Drawing for the job (mm, zero at the part's lowest x, y, z). Give positions to 0.01 mm unless a question says otherwise; leave off trailing zeros. Loops run counter-clockwise (first coordinate to the right, second up) from the corner with the lowest first, then second, coordinate; pieces in that order, holes last. Notation, with made-up numbers: (-20, -5.5) -> (38, -5.5) arc R20 cw to (38, 26.5) -> close; hole circle Ø10 at (6.5, 7). An arc over 180 degrees is marked (long way). Answer in a Markdown table with one row per item. Add a question column.
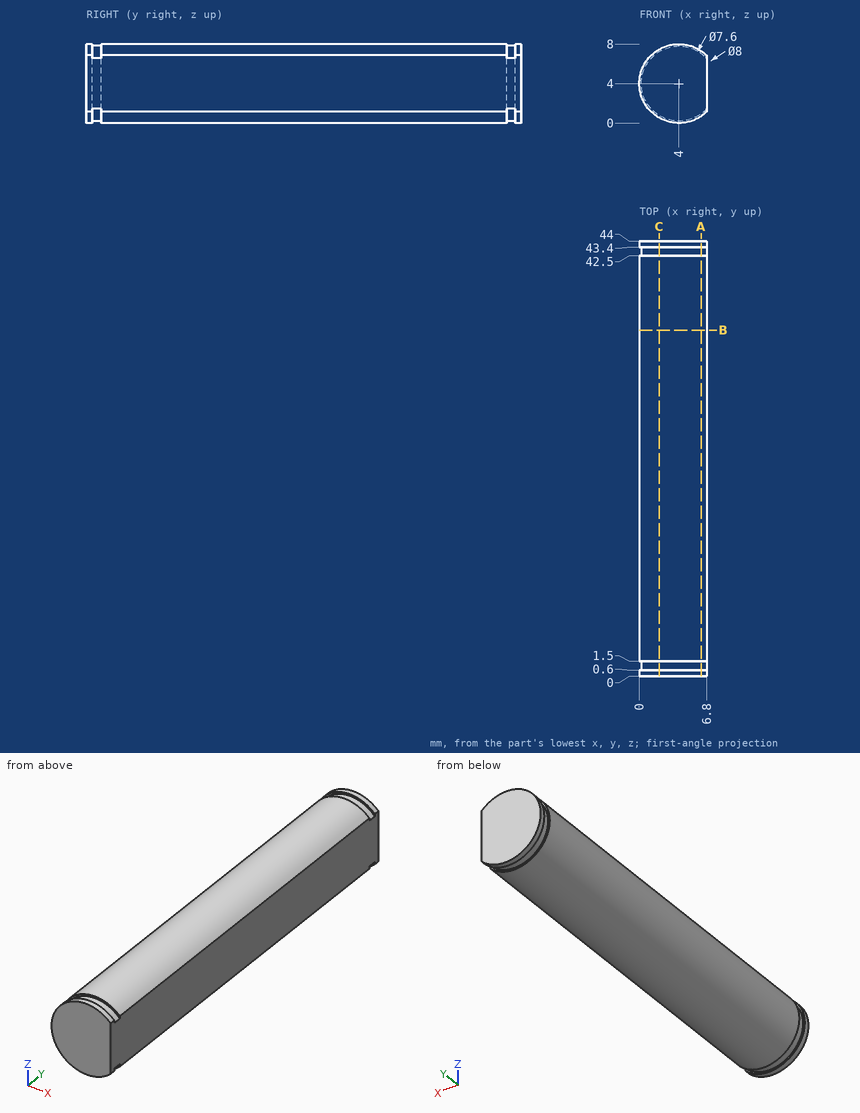
(1) Saw through at C-C, the plane x = 2. List the corners of the cut face in (y, z).
(2) Wall check: line 1 along X through (y, z) = (41.5, 3.75); line 2 along Z through (x, y) = (4.25, 7.5); line 3 along X through (y, z) = (40.5, 2). Give the ranges that are in metal, low to high. Write a range as from..to.
(3) Saw through at A-A, the plane x = 6.25. List the corners of the cut face in (y, z), then the cut area to 3 significant figures.
(4) Saw through at B-B, the plane y = 35. List the corners of the cut face in (x, z), then the cut area to 3 significant figures.
Worked answers:
| question | item | result |
|---|---|---|
| 1 | outline | (0, 0.54) -> (0.6, 0.54) -> (0.6, 0.77) -> (1.5, 0.77) -> (1.5, 0.54) -> (42.5, 0.54) -> (42.5, 0.77) -> (43.4, 0.77) -> (43.4, 0.54) -> (44, 0.54) -> (44, 7.46) -> (43.4, 7.46) -> (43.4, 7.23) -> (42.5, 7.23) -> (42.5, 7.46) -> (1.5, 7.46) -> (1.5, 7.23) -> (0.6, 7.23) -> (0.6, 7.46) -> (0, 7.46) -> close |
| 2 | line 1 | 0.01..6.8 |
| 2 | line 2 | 0.01..7.99 |
| 2 | line 3 | 0.54..6.8 |
| 3 | outline | (0, 0.69) -> (0.6, 0.69) -> (0.6, 0.94) -> (1.5, 0.94) -> (1.5, 0.69) -> (42.5, 0.69) -> (42.5, 0.94) -> (43.4, 0.94) -> (43.4, 0.69) -> (44, 0.69) -> (44, 7.31) -> (43.4, 7.31) -> (43.4, 7.06) -> (42.5, 7.06) -> (42.5, 7.31) -> (1.5, 7.31) -> (1.5, 7.06) -> (0.6, 7.06) -> (0.6, 7.31) -> (0, 7.31) -> close |
| 3 | area | 290 mm^2 |
| 4 | outline | (6.8, 1.14) -> (6.8, 6.86) arc R4 ccw (long way) to start |
| 4 | area | 45.5 mm^2 |
